Check sheet for the modelled part. Datum: model origin and axes. Units: mm. A direction names the side the tool comes from. Give positions to 0.01 mm unless a question says otherwise; leave off trailing zeros. Order: outer loops, then holes, each group sorted by start corner. A loop starts at its lowest first (then second) coordinate and runs counter-clockwise, first axis right, second up.
from build123d import *

# Parameters (mm, degrees)
SKETCH1_R           = 62
SKETCH1_R_2         = 5.5
SKETCH1_R_3         = 29
BOSS_EXTRUDE1_DEPTH = 10
SKETCH2_R           = 40
SKETCH2_R_2         = 29
SKETCH2_R_3         = 3
BOSS_EXTRUDE2_DEPTH = 20
BOSS_EXTRUDE3_START = -5
SKETCH3_R           = 3
BOSS_EXTRUDE3_DEPTH = 5
CHAMFER2_SIZE       = 5
CHAMFER3_SIZE       = 1
SKETCH6_R           = 29
SKETCH6_R_2         = 26
BOSS_EXTRUDE4_DEPTH = 13
CHAMFER4_SIZE       = 10


with BuildPart() as part:
    # Sketch1 → Boss-Extrude1 (new body)
    with BuildSketch(Plane(origin=(0, 0, 0), x_dir=(1, 0, 0), z_dir=(0, 1, 0))):
        Circle(SKETCH1_R)
        with Locations((51, 0)):
            Circle(SKETCH1_R_2, mode=Mode.SUBTRACT)
        with Locations((41.259866713, -29.977047867)):
            Circle(SKETCH1_R_2, mode=Mode.SUBTRACT)
        with Locations((15.759866713, -48.503882331)):
            Circle(SKETCH1_R_2, mode=Mode.SUBTRACT)
        with Locations((-15.759866713, -48.503882331)):
            Circle(SKETCH1_R_2, mode=Mode.SUBTRACT)
        with Locations((-41.259866713, -29.977047867)):
            Circle(SKETCH1_R_2, mode=Mode.SUBTRACT)
        with Locations((-51, 0)):
            Circle(SKETCH1_R_2, mode=Mode.SUBTRACT)
        with Locations((-41.259866713, 29.977047867)):
            Circle(SKETCH1_R_2, mode=Mode.SUBTRACT)
        with Locations((-15.759866713, 48.503882331)):
            Circle(SKETCH1_R_2, mode=Mode.SUBTRACT)
        with Locations((15.759866713, 48.503882331)):
            Circle(SKETCH1_R_2, mode=Mode.SUBTRACT)
        with Locations((41.259866713, 29.977047867)):
            Circle(SKETCH1_R_2, mode=Mode.SUBTRACT)
        Circle(SKETCH1_R_3, mode=Mode.SUBTRACT)
    extrude(amount=BOSS_EXTRUDE1_DEPTH)

    # Sketch2 → Boss-Extrude2 (add)
    with BuildSketch(Plane(origin=(0, 0, 0), x_dir=(1, 0, 0), z_dir=(0, 1, 0))):
        Circle(SKETCH2_R)
        Circle(SKETCH2_R_2, mode=Mode.SUBTRACT)
        with Locations((35, 0)):
            Circle(SKETCH2_R_3, mode=Mode.SUBTRACT)
        with Locations((28.315594803, -20.57248383)):
            Circle(SKETCH2_R_3, mode=Mode.SUBTRACT)
        with Locations((10.815594803, -33.28697807)):
            Circle(SKETCH2_R_3, mode=Mode.SUBTRACT)
        with Locations((-10.815594803, -33.28697807)):
            Circle(SKETCH2_R_3, mode=Mode.SUBTRACT)
        with Locations((-28.315594803, -20.57248383)):
            Circle(SKETCH2_R_3, mode=Mode.SUBTRACT)
        with Locations((-35, 0)):
            Circle(SKETCH2_R_3, mode=Mode.SUBTRACT)
        with Locations((-28.315594803, 20.57248383)):
            Circle(SKETCH2_R_3, mode=Mode.SUBTRACT)
        with Locations((-10.815594803, 33.28697807)):
            Circle(SKETCH2_R_3, mode=Mode.SUBTRACT)
        with Locations((10.815594803, 33.28697807)):
            Circle(SKETCH2_R_3, mode=Mode.SUBTRACT)
        with Locations((28.315594803, 20.57248383)):
            Circle(SKETCH2_R_3, mode=Mode.SUBTRACT)
    extrude(amount=BOSS_EXTRUDE2_DEPTH)

    # Sketch3 → Boss-Extrude3 (add)
    with BuildSketch(Plane(origin=(0, 20, 0), x_dir=(1, 0, 0), z_dir=(0, 1, 0)).offset(BOSS_EXTRUDE3_START)):
        with Locations((-28.315594803, -20.57248383)):
            Circle(SKETCH3_R)
        with Locations((-35, 0)):
            Circle(SKETCH3_R)
        with Locations((-28.315594803, 20.57248383)):
            Circle(SKETCH3_R)
        with Locations((-10.815594803, 33.28697807)):
            Circle(SKETCH3_R)
        with Locations((10.815594803, 33.28697807)):
            Circle(SKETCH3_R)
        with Locations((28.315594803, 20.57248383)):
            Circle(SKETCH3_R)
        with Locations((35, 0)):
            Circle(SKETCH3_R)
        with Locations((28.315594803, -20.57248383)):
            Circle(SKETCH3_R)
        with Locations((10.815594803, -33.28697807)):
            Circle(SKETCH3_R)
        with Locations((-10.815594803, -33.28697807)):
            Circle(SKETCH3_R)
    extrude(amount=-BOSS_EXTRUDE3_DEPTH)

    # Chamfer2
    chamfer2_edges = [part.edges().sort_by_distance(p)[0] for p in [
        (-62, 10, 0),
    ]]
    chamfer(chamfer2_edges, length=CHAMFER2_SIZE)

    # Chamfer3
    chamfer3_edges = [part.edges().sort_by_distance(p)[0] for p in [
        (10.259866713, 0, -48.503882331),
        (-21.259866713, 0, -48.503882331),
        (-46.759866713, 0, -29.977047867),
        (-56.5, 0, 0),
        (-46.759866713, 0, 29.977047867),
        (-21.259866713, 0, 48.503882331),
        (10.259866713, 0, 48.503882331),
        (35.759866713, 0, 29.977047867),
        (45.5, 0, 0),
        (35.759866713, 0, -29.977047867),
    ]]
    chamfer(chamfer3_edges, length=CHAMFER3_SIZE)

    # Sketch6 → Boss-Extrude4 (add)
    with BuildSketch(Plane.XZ):
        Circle(SKETCH6_R)
        Circle(SKETCH6_R_2, mode=Mode.SUBTRACT)
    extrude(amount=-BOSS_EXTRUDE4_DEPTH)

    # Chamfer4
    chamfer4_edges = [part.edges().sort_by_distance(p)[0] for p in [
        (-26, 0, 0),
    ]]
    chamfer(chamfer4_edges, length=CHAMFER4_SIZE)


solid = part.part
1) Depth check by flat-ended pin: pin 1 Ø12.5 at (x, z) = (41.26, 29.98) entering from +Y; pin 2 Ø3.5 at (x, z) = (35, 0) entering from +Y; pin 3 Ø6.5 at (x, z) = (29.5, 21) entering from +Y; pin 4 Ø2 at (x, z) = (-17, -22.5) entering from -Y. Enter the tip coordinate at first touch or a pass-through.
Recorded:
pin 1: stops at y = 10
pin 2: stops at y = 15
pin 3: stops at y = 20
pin 4: stops at y = 6.8
2) Set-up check for faces 1 (the face through (-8.071, 2.465, -61.472)), 2 (the face through (28, 15, 21)): record each of +Z, -Z, +X, -X, +Y, -Y from which the full face is reachable in a straight line by a thin tool's end or side.
Recorded:
face 1: +Y, -Y
face 2: +Y
3) Section check B-B, the plane z = 0. State how many separate pieces and enclosed holes the cut face has, then the cut area to 3 significant figures.
Recorded:
separate pieces: 4
enclosed holes: 0
area: 551 mm2
4) Draft check along X on faces 3 (the face through (27, 0, -27)), 4 (the face through (-7.954, 17.465, -34.188)), 5 (the face through (-8.67, 14.93, 39.05)). Enter one of: +X half, -X half, draft (parallel to the pull), parting line (faces both ways), or undercut.
Recorded:
face 3: draft
face 4: undercut
face 5: parting line
5) Section check A-A, the plane x = 0. Record the cut outline in (y, z), then the cut area to 3 significant figures.
Recorded:
outline: (0, -62) - (5, -62) - (10, -57) - (10, -40) - (20, -40) - (20, -29) - (13, -29) - (13, -26) - (10, -26) - (0, -36) - close; (0, 36) - (10, 26) - (13, 26) - (13, 29) - (20, 29) - (20, 40) - (10, 40) - (10, 57) - (5, 62) - (0, 62) - close
area: 833 mm2
6) Material ranges on L1, parallel to Y at x = 51.5, z = 24; L2, parallel to Z at x = 15, y = 4.25; L3, parallel to X at y = 7.5, z = -29, recorded low to high.
Recorded:
L1: y = 0 to 10
L2: z = -60.16 to -53.95, -43.06 to -27.98, 27.98 to 43.06, 53.95 to 60.16
L3: x = -51.95 to -46.67, -35.85 to 35.85, 46.67 to 51.95
